Autodesk Inventor part; units mm, degrees
ref_plane "YZ Plane" through (0, 0, 0) normal (1, 0, 0) x (0, 1, 0)
ref_plane "XZ Plane" through (0, 0, 0) normal (0, 1, 0) x (-1, 0, 0)
ref_plane "XY Plane" through (0, 0, 0) normal (0, 0, 1) x (1, 0, 0)
sketch "Sketch1" plane through (0, 0, 0) normal (0, 1, 0) x (-1, 0, 0)
  circle A0 centre (0, 0) radius 18.415
  dimension "d0" = 36.83
extrude "Extrusion1" add sketch "Sketch1" along normal blind 52.832
sketch "Sketch2" plane through (0, 52.832, 0) normal (0, 1, 0) x (1, 0, 0)
  circle A0 centre (0, 6.8072) radius 5.6642
  line L0 (-18.3795, 1.143) -> (18.3795, 1.143) construction
  circle A1 centre (0, 0) radius 18.415
  line L1 (-28.9381, -18.415) -> (33.3416, -18.415) construction
  circle A2 centre (0, 0) radius 18.415
  dimension "d3" = 11.3284
  dimension "d10" = 19.558
extrude "Extrusion2" add sketch "Sketch2" along normal blind 5.08 contours A0
sketch "Sketch3" plane through (0, 57.912, -6.8072) normal (0, 1, 0) x (1, 0, 0)
  circle A0 centre (0, 0) radius 2.921
  point P0 (0, -6.8072)
  dimension "d6" = 5.842
extrude "Extrusion3" add sketch "Sketch3" along normal blind 19.558
sketch "Sketch4" plane through (0, 52.832, 0) normal (0, 1, 0) x (1, 0, 0)
  circle A0 centre (-7.747, 13.4182) radius 1.143
  circle A1 centre (0, 6.8072) radius 5.6642
  circle A2 centre (0, 0) radius 18.415
  circle A3 centre (-15.494, 0) radius 1.143
  circle A4 centre (-7.747, -13.4182) radius 1.143
  circle A5 centre (7.747, -13.4182) radius 1.143
  circle A6 centre (15.494, 0) radius 1.143
  circle A7 centre (7.747, 13.4182) radius 1.143
  circle A8 centre (0, 0) radius 18.415
  line L0 (0, 0) -> (-16.637, 0) construction
  line L1 (-18.415, 3.3425) -> (-18.415, -3.4032) construction
  dimension "d11" = 2.286
  dimension "d14" = 360
  dimension "d16" = 1.778
extrude "Extrusion4" cut sketch "Sketch4" against normal blind 7.62 contours A0 | A3 | A4 | A5 | A6 | A7
properties part number "DC 12V 200RPM"
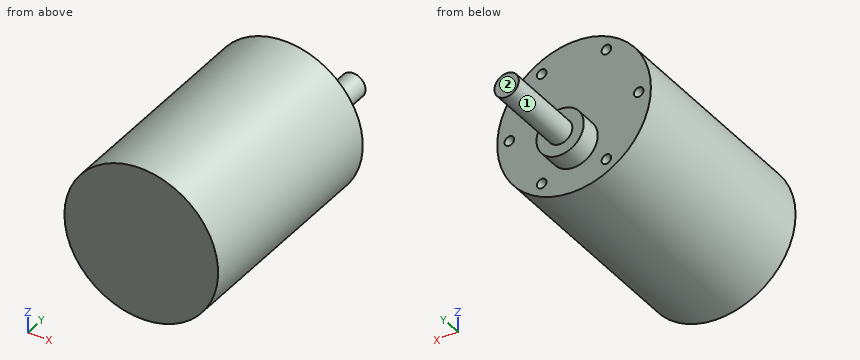
Geometry check sheet. Reference: the model listing, model coordinates, mm. Face numbers are marked on the shaded views. A direction names the side the tool comes from. Coordinates: 2 decimals unless noted, no trailing zeros. Order: outer loops, then holes, each group sorted by start corner. A loop starts at its lowest first (then second) coordinate and runs counter-clockwise, first axis right, second up. Notation, with made-up numbers: M 72.25,-12.5 L 93.25,-12.5 A10 ccw 93.25,0.5 Z; hole C 46,59 d10. An arc over 180 degrees is marked long. Use CSV: the item, a comma, the result in double quotes.
Item 1: Cross-section at D-D on y = 64. Record the cut outline in (x, z), then the cut area to 3 significant figures.
Returned:
outline,"C 0,-6.81 d5.84"
area,"26.8 mm2"
Item 2: Gauge pin test, flat ends, axial feed: pin 1 Ø4 at (y, z) = (39.5, -13.5) entering from -X; pin 2 Ø2.5 at (x, z) = (15.5, 0.5) entering from +Y; pin 3 Ø1.1 at (x, z) = (8, 13.5) entering from +Y. Record the tip position at first contact, or that the pin passes through.
Returned:
pin 1,"stops at x = -14.38"
pin 2,"stops at y = 52.83"
pin 3,"stops at y = 45.21"
Item 3: Cross-section at A-A on z = 0. Record the cut outline in (x, y) (3 decimals), then the cut area to 3 significant figures.
Returned:
outline,"M -18.415,0 L 18.415,0 L 18.415,52.832 L 16.637,52.832 L 16.637,45.212 L 14.351,45.212 L 14.351,52.832 L -14.351,52.832 L -14.351,45.212 L -16.637,45.212 L -16.637,52.832 L -18.415,52.832 Z"
area,"1,910 mm2"
Item 4: Tool access check on the marked faces 1 and 2. Record the directions out of +Z, -Z, +X, -X, +Y, -Y that give a thin tool (end or side, any length) a straight path to the whole face; none if there is none.
Returned:
face 1,"+Y"
face 2,"+Z, -Z, +X, -X, +Y"
Item 5: Cross-section at C-C on y = 37.5. Record the cut outline in (x, z) (3 decimals).
Returned:
outline,"C 0,0 d36.83"
Item 6: Cross-section at B-B on x = 0. Record the cut outline in (y, z) (3 decimals), then the cut area to 3 significant figures.
Returned:
outline,"M 0,-18.415 L 52.832,-18.415 L 52.832,-12.471 L 57.912,-12.471 L 57.912,-9.728 L 77.47,-9.728 L 77.47,-3.886 L 57.912,-3.886 L 57.912,-1.143 L 52.832,-1.143 L 52.832,18.415 L 0,18.415 Z"
area,"2,120 mm2"
Item 7: Thickness scan on line 1 along Y through (x, z) = (-13.5, 7); line 2 along Z through (x, y) = (0.5, 9); line 3 along Z through (x, y) = (15.5, 50.5). Record the ranges inside material, lowest first.
Returned:
line 1,"y = 0 to 52.83"
line 2,"z = -18.41 to 18.41"
line 3,"z = -9.94 to -1.14, 1.14 to 9.94"
